Read the model definition and answer for the solid it produces. Units are mm, in the model's axes. A direction names the side the tool comes from. Coordinates: 2 decimals unless noted, no trailing zeros. Write each loop counter-clockwise with the first axis right and the second up, starting at its lowest first coordinate (ties: lowest second). Pieces come first, ordered by that corner, then holes. Notation, with made-up numbers: (41.25, -17.75) -> (69.25, -17.75) arc R29 cw to (69.25, 19.25) -> close; hole circle Ø4 at (26, 22.5). An arc over 180 degrees is marked (long way). Write item = value, one per line. Start each with the question number.
1) Section D-D (x = 13) is taken. Determine the outline of the cut face in (y, z) (3 decimals).
2) For a pull along Z with two mould halves and no side action, classify faces 1 (the face through (2.25, 21.45, -0.17)), 2 (the face through (0.254, 14, 1.2)), 3 (the face through (-15.621, 13, 0)), 4 (the face through (6, 13, 6.35)) as released by +Z, released by -Z, zero draft, split by the parting line, or undercut.
3) Find the intervals of material crossed by line 1 along Y through (x, z) = (3.05, 0); line 2 along Y through (x, z) = (12, 0.5); line 3 along Y through (x, z) = (3, -2.5), in increasing order. Write a range as from..to.
4) A flat-ended cylindrical pin translates along its axis: pin 1 Ø1.9 at (y, z) = (25, 1.5) entering from -X. Find the tip coordinate at first contact, or state that the pin passes through.
5) Section B-B (x = 6.5) is taken. Determine the outline of the cut face in (y, z) (3 decimals).
6) A tool of negligible diameter and unlimited length cuts with its end or side. For faces 5 (the face through (0.127, 0.5, 4.8)), 6 (the face through (0.127, 25, -5)), 7 (the face through (0.127, 0.6, -4.8)), from which of +Z, -Z, +X, -X, +Y, -Y can it reach the whole face along a straight path? Write none if from no direction.
from build123d import *

# Parameters (mm, degrees)
BOSS_EXTRUDE1_DEPTH = 25.4
SKETCH2_R           = 6.35
SKETCH2_R_2         = 4.7625
BOSS_EXTRUDE2_DEPTH = 3.175
SKETCH3_R           = 4.7625
CUT_EXTRUDE1_DEPTH  = 26.19375
SKETCH4_R           = 5.55625
CUT_EXTRUDE2_DEPTH  = 0.254
SKETCH5_R           = 1.5875
BOSS_EXTRUDE3_DEPTH = 15.875
SKETCH6_R           = 0.79375
CUT_EXTRUDE3_DEPTH  = 4.572
CUT_EXTRUDE4_DEPTH  = 0.127


with BuildPart() as part:
    # Sketch1 → Boss-Extrude1 (new body)
    with BuildSketch(Plane(origin=(0, 0, 0), x_dir=(1, 0, 0), z_dir=(0, 1, 0))):
        Polygon((0, -6.35), (0, 6.35), (12.155256121, 6.35), (15.875, 2.630256121), (15.875, -2.630256121), (12.155256121, -6.35), align=None)
    extrude(amount=BOSS_EXTRUDE1_DEPTH)

    # Sketch2 → Boss-Extrude2 (add)
    with BuildSketch(Plane.XZ):
        with Locations((9.525, 0)):
            Circle(SKETCH2_R)
        with Locations((9.525, 0)):
            Circle(SKETCH2_R_2, mode=Mode.SUBTRACT)
    extrude(amount=BOSS_EXTRUDE2_DEPTH)

    # Sketch3 → Cut-Extrude1 (cut)
    with BuildSketch(Plane.XZ.offset(3.175)):
        with Locations((9.525, 0)):
            Circle(SKETCH3_R)
    extrude(amount=-CUT_EXTRUDE1_DEPTH, mode=Mode.SUBTRACT)

    # Sketch4 → Cut-Extrude2 (cut)
    with BuildSketch(Plane.ZY):
        with Locations((0, 12.7)):
            Circle(SKETCH4_R)
    extrude(amount=-CUT_EXTRUDE2_DEPTH, mode=Mode.SUBTRACT)

    # Sketch5 → Boss-Extrude3 (add)
    with BuildSketch(Plane.ZY.offset(-0.254)):
        with Locations((0, 12.7)):
            Circle(SKETCH5_R)
    extrude(amount=BOSS_EXTRUDE3_DEPTH)

    # Sketch6 → Cut-Extrude3 (cut)
    with BuildSketch(Plane.ZY):
        with Locations((0, 22.225)):
            Circle(SKETCH6_R)
    extrude(amount=-CUT_EXTRUDE3_DEPTH, mode=Mode.SUBTRACT)

    # Sketch7 → Cut-Extrude4 (cut)
    with BuildSketch(Plane.ZY):
        with BuildLine():
            ThreePointArc((0, 25.4), (3.287001873, 24.967257994), (6.35, 23.698522628))
            Line((6.35, 23.698522628), (6.35, 25.4))
            Line((6.35, 25.4), (0, 25.4))
        make_face()
        with BuildLine():
            Line((-6.35, 25.4), (-6.35, 23.698522628))
            ThreePointArc((-6.35, 23.698522628), (-3.287001873, 24.967257994), (0, 25.4))
            Line((0, 25.4), (-6.35, 25.4))
        make_face()
        with BuildLine():
            Line((-6.35, 1.701477372), (-6.35, 0))
            Line((-6.35, 0), (0, 0))
            ThreePointArc((0, 0), (-3.287001873, 0.432742006), (-6.35, 1.701477372))
        make_face()
        with BuildLine():
            ThreePointArc((6.35, 1.701477372), (3.287001873, 0.432742006), (0, 0))
            Line((0, 0), (6.35, 0))
            Line((6.35, 0), (6.35, 1.701477372))
        make_face()
    extrude(amount=-CUT_EXTRUDE4_DEPTH, mode=Mode.SUBTRACT)


solid = part.part
Answer key:
q1.outline = (-3.175, -5.315) -> (0, -5.315) -> (0, -5.505) -> (25.4, -5.505) -> (25.4, 5.505) -> (0, 5.505) -> (0, 5.315) -> (-3.175, 5.315) -> (-3.175, 3.257) -> (23.019, 3.257) -> (23.019, -3.257) -> (-3.175, -3.257) -> close
q2.face_1 = undercut
q2.face_2 = undercut
q2.face_3 = zero draft
q2.face_4 = released by +Z
q3.line_1 = 0..21.43, 23.02..25.4
q3.line_2 = 23.02..25.4
q3.line_3 = 0..25.4
q4.pin_1 = 0
q5.outline = (-3.175, -5.583) -> (0, -5.583) -> (0, -6.35) -> (25.4, -6.35) -> (25.4, 6.35) -> (0, 6.35) -> (0, 5.583) -> (-3.175, 5.583) -> (-3.175, 3.678) -> (23.019, 3.678) -> (23.019, -3.678) -> (-3.175, -3.678) -> close
q6.face_5 = +Z, -X, -Y
q6.face_6 = -Z, -X, +Y
q6.face_7 = -Z, -X, -Y
